Model file for the job. Use its own axes, mm. A direction names the side the tool comes from. Coordinates: 2 decimals unless noted, no trailing zeros. Order: outer loops, then holes, each group sorted by start corner. A loop starts at its lowest first (then second) coordinate and runs counter-clockwise, first axis right, second up. Notation, with made-up numbers: M 58.5,5 L 80.5,5 A9 cw 80.5,16 Z; hole C 64.5,10.25 d1. An arc over 180 degrees is marked long. Return JSON: item names as keys, results as strings.
```python
from build123d import *

# Parameters (mm, degrees)
F0_W     = 880
F0_H     = 690
F1_DEPTH = 210
F2_W     = 880
F2_H     = 210
F2_W_2   = 40
F2_H_2   = 40
F3_DEPTH = 80
F4_W     = 844
F4_H     = 278
F5_DEPTH = 207


# Not quite as in the source:
# - a feature names something its author has since deleted; it is built from what else it names


with BuildPart() as f1:
    # F0 (on Front) → F1 (new body)
    with BuildSketch(Plane.XZ):
        with Locations((402.0964676142, 312.2104381025)):
            Rectangle(F0_W, F0_H)
    extrude(amount=F1_DEPTH)

    # F2 (on face) → F3 (cut)
    with BuildSketch(Plane(origin=(0, 0, -32.7895618975), x_dir=(1, 0, 0), z_dir=(0, 0, -1))):
        with Locations((402.0964676142, 105)):
            Rectangle(F2_W, F2_H)
        with Locations((12.0964676142, 50)):
            Rectangle(F2_W_2, F2_H_2, mode=Mode.SUBTRACT)
        with Locations((792.0964676142, 50)):
            Rectangle(F2_W_2, F2_H_2, mode=Mode.SUBTRACT)
        with Locations((12.0964676142, 160)):
            Rectangle(F2_W_2, F2_H_2, mode=Mode.SUBTRACT)
        with Locations((792.0964676142, 160)):
            Rectangle(F2_W_2, F2_H_2, mode=Mode.SUBTRACT)
    extrude(amount=-F3_DEPTH, mode=Mode.SUBTRACT)

    # F4 (on face) → F5 (cut, through all)
    with BuildSketch(Plane.XZ.offset(210)):
        with Locations((402.0964676142, 500.2104381025)):
            Rectangle(F4_W, F4_H)
        with Locations((402.0964676142, 204.2104381025)):
            Rectangle(F4_W, F4_H)
    extrude(amount=-F5_DEPTH, mode=Mode.SUBTRACT)


solid = f1.part
```
Item 1: Saw through at A-A (y = -157.5). Write the cut outline in (x, z).
Check result:
{"outline": "M -37.9,47.21 L -7.9,47.21 L -7.9,-32.79 L 32.1,-32.79 L 32.1,47.21 L 772.1,47.21 L 772.1,-32.79 L 812.1,-32.79 L 812.1,47.21 L 842.1,47.21 L 842.1,657.21 L -37.9,657.21 Z; hole M -19.9,65.21 L 824.1,65.21 L 824.1,343.21 L -19.9,343.21 Z; hole M -19.9,361.21 L 824.1,361.21 L 824.1,639.21 L -19.9,639.21 Z"}
Item 2: 3-axis set-ups, long thin cutter, end or side, ignore diameter. For faces 4 (the flat face through (396, -108, 361.21)), 5 (the flat face through (12, -180, 7)), 6 (the flat face through (812.096, -160, 7)): which of +Z, -Z, +X, -X, +Y, -Y reach the whole face in a straight line?
Check result:
{"face 4": "-Y", "face 5": "-Z, +X, -X, -Y", "face 6": "-Z, +X, +Y, -Y"}
Item 3: Drop flat-ended pins along their axis: pin 1 Ø12 at (x, y) = (504.5, -117.5) entering from -Z; pin 2 Ø20 at (y, z) = (-51.5, -12) entering from -X; pin 3 Ø12 at (x, z) = (12.5, 21.5) entering from +Y. Give the stop position or say it passes through.
Check result:
{"pin 1": "stops at z = 47.21", "pin 2": "stops at x = -7.9", "pin 3": "stops at y = -30"}
Item 4: Pull direction Y, two halves, no side cores. Call faces 1 (the flat face through (12, -140, 7)), 2 (the flat face through (792, -180, 7)), 3 (the flat face through (32.096, -50, 7)): +Y half, -Y half, draft (parallel to the pull), parting line (faces both ways), or undercut.
Check result:
{"face 1": "undercut", "face 2": "-Y half", "face 3": "draft"}
Item 5: Wall check: line 1 (Z direction, x = 371, y = -96); line 2 (X direction, y = -161, z = 161); line 3 (Y direction, x = 777.5, z = 10). Give the ranges that are in metal, low to high.
Check result:
{"line 1": "z = 47.21 to 65.21, 343.21 to 361.21, 639.21 to 657.21", "line 2": "x = -37.9 to -19.9, 824.1 to 842.1", "line 3": "y = -180 to -140, -70 to -30"}
Item 6: Saw through at C-C (x = 668). Write the cut outline in (y, z).
Check result:
{"outline": "M -210,47.21 L 0,47.21 L 0,657.21 L -210,657.21 L -210,639.21 L -3,639.21 L -3,361.21 L -210,361.21 L -210,343.21 L -3,343.21 L -3,65.21 L -210,65.21 Z"}
Item 7: Saw through at B-B (z = 261). Write the cut outline in (x, y).
Check result:
{"outline": "M -37.9,-210 L -19.9,-210 L -19.9,-3 L 824.1,-3 L 824.1,-210 L 842.1,-210 L 842.1,0 L -37.9,0 Z"}
